```python
from build123d import *

# Parameters (mm, degrees)
PAD007_DEPTH    = 1.5
PAD008_DEPTH    = 0.5
SKETCH012_W     = 5
SKETCH012_H     = 2.5
SKETCH012_W_2   = 7.5
PAD009_DEPTH    = 0.8
SKETCH013_W     = 7.5
SKETCH013_H     = 3
PAD010_DEPTH    = 0.5
POCKET003_DEPTH = 0.5
POCKET004_DEPTH = 2
SKETCH021_W     = 5
SKETCH021_H     = 8
PAD013_DEPTH    = 3.2
SKETCH024_R     = 2.65
POCKET007_DEPTH = 5.201


with BuildPart() as part:
    # Sketch010 → Pad007 (new body)
    with BuildSketch(Plane.XY.offset(-19)):
        with BuildLine():
            Line((-29.25, 13), (29.25, 13))
            ThreePointArc((33, 9.25), (31.9016504294, 11.9016504294), (29.25, 13))
            Line((33, 9.25), (33, -9.25))
            ThreePointArc((29.25, -13), (31.9016504295, -11.9016504294), (33, -9.25))
            Line((29.25, -13), (-29.25, -13))
            ThreePointArc((-33, -9.25), (-31.9016504294, -11.9016504295), (-29.25, -13))
            Line((-33, -9.25), (-33, 9.25))
            ThreePointArc((-29.25, 13), (-31.9016504294, 11.9016504294), (-33, 9.25))
        make_face()
    extrude(amount=PAD007_DEPTH)

    # Sketch011 → Pad008 (new body)
    with BuildSketch(Plane.XY.offset(-17.5)):
        with BuildLine():
            Line((-29.05, 11.3), (29.05, 11.3))
            ThreePointArc((31.3, 9.05), (30.6409902577, 10.6409902577), (29.05, 11.3))
            Line((31.3, 9.05), (31.3, -9.05))
            ThreePointArc((29.05, -11.3), (30.6409902577, -10.6409902577), (31.3, -9.05))
            Line((29.05, -11.3), (-29.05, -11.3))
            ThreePointArc((-31.3, -9.05), (-30.6409902577, -10.6409902577), (-29.05, -11.3))
            Line((-31.3, -9.05), (-31.3, 9.05))
            ThreePointArc((-29.05, 11.3), (-30.6409902577, 10.6409902577), (-31.3, 9.05))
        make_face()
    extrude(amount=PAD008_DEPTH)

    # Sketch012 → Pad009 (new body)
    with BuildSketch(Plane.XY.offset(-17)):
        with Locations((-10.5, 10.55)):
            Rectangle(SKETCH012_W, SKETCH012_H)
        with Locations((10.5, 10.55)):
            Rectangle(SKETCH012_W, SKETCH012_H)
        with Locations((0, -9.75)):
            Rectangle(SKETCH012_W_2, SKETCH012_H)
    extrude(amount=PAD009_DEPTH)

    # Sketch013 → Pad010 (new body)
    with BuildSketch(Plane.XY.offset(-16.2)):
        with Locations((0, -10)):
            Rectangle(SKETCH013_W, SKETCH013_H)
    extrude(amount=PAD010_DEPTH)

    # Sketch016 → Pocket003 (cut)
    with BuildSketch(Plane.XY.offset(-17)):
        with BuildLine():
            ThreePointArc((28.0000015561, -6.5), (26.2322341473, -7.2322319467), (25.5, -8.9999984439))
            ThreePointArc((23.2000163651, -11.3), (24.8263541015, -10.6263414294), (25.5, -8.999998444))
            Line((23.2000163651, -11.5), (23.2000163651, -11.3))
            Line((31.5, -11.5), (23.2000163651, -11.5))
            Line((31.5, -3.2000163651), (31.5, -11.5))
            Line((31.3, -3.2000163651), (31.5, -3.2000163651))
            ThreePointArc((28.0000015561, -6.5), (30.3334480205, -5.5334584921), (31.3, -3.2000163651))
        make_face()
        with BuildLine():
            Line((-23.2000163651, 11.3), (-23.2000163651, 11.5))
            Line((-23.2000163651, 11.5), (-31.5, 11.5))
            Line((-31.5, 11.5), (-31.5, 3.2000163651))
            Line((-31.5, 3.2000163651), (-31.3, 3.2000163651))
            ThreePointArc((-28.000005004, 6.5), (-30.3334514906, 5.5334595241), (-31.3, 3.2000163651))
            ThreePointArc((-28.000005004, 6.5), (-26.2322365854, 7.2322295087), (-25.5, 8.999994996))
            ThreePointArc((-23.2000163651, 11.3), (-24.8263548156, 10.6263397054), (-25.5, 8.999994996))
        make_face()
    extrude(amount=-POCKET003_DEPTH, mode=Mode.SUBTRACT)

    # Sketch017 → Pocket004 (cut)
    with BuildSketch(Plane.XY.offset(-17)):
        with BuildLine():
            ThreePointArc((-24, -6.1), (-25.2, -7.3), (-24, -8.5))
            Line((-24, -8.5), (24, -8.5))
            ThreePointArc((24, -8.5), (25.2, -7.3), (24, -6.1))
            Line((-24, -6.1), (24, -6.1))
        make_face()
    extrude(amount=-POCKET004_DEPTH, mode=Mode.SUBTRACT)

    # Sketch021 → Pad013 (new body)
    with BuildSketch(Plane.XY.offset(-17)):
        with Locations((28.8, 0)):
            Rectangle(SKETCH021_W, SKETCH021_H)
    extrude(amount=PAD013_DEPTH)

    # Sketch024 → Pocket007 (cut, through all)
    with BuildSketch(Plane(origin=(0, 0, -19), x_dir=(1, 0, 0), z_dir=(0, 0, -1))):
        with Locations((-20, -9)):
            Circle(SKETCH024_R)
    extrude(amount=-POCKET007_DEPTH, mode=Mode.SUBTRACT)


solid = part.part
```
Could you check a few things on this model? Use its own coordinates, in mm. A direction names the side the tool comes from. Round coordinates to 2 decimals unless told otherwise and drop trailing zeros. Loops run counter-clockwise (first coordinate to the right, second up) from the corner with the lowest first, then second, coordinate; pieces in that order, holes last. Notation, with made-up numbers: (44.25, -24) - (85.25, -24) arc R17 cw to (85.25, -17) - close; hole circle Ø11 at (-32.75, 88.5). An arc over 180 degrees is marked (long way). Answer in a Markdown table with one row per item. Add a question column.
(1) If we section it at C-C (y = -7.3): Please give me the cut outline in (x, z).
(2) If we mould it in two halves opening along X, with no side actions, what happens to faces 1 (the face through (-26.252, 7.213, -17.246)), 2 (the face through (0, -8.5, -18)), 3 (the face through (0, 13, -18))? For each: pulls with the +X half, pulls with the -X half, needs draft (parallel to the pull), parting line crosses it, or undercut.
(3) I'm going to push flat-ended pins straight in: pin 1 (8 mm diameter, centred on x = 7.5, y = -0.5, fed in from +Z); pin 2 (0.6 mm diameter, centred on x = 1.5, z = -16, fed in from -Y); pin 3 (1 mm diameter, centred on y = -2, z = -16.5, fed in from +X). Where does each tip first touch, or does it pass through?
(4) If we section it at D-D (x = 18): Please give me the cut outline in (y, z), plus the area to 3 significant figures.
(5) If we section it at B-B (x = -20): Please give me the cut outline in (y, z).
(6) If we section it at A-A (x = -11): Please give me the cut outline in (y, z), plus the area to 3 significant figures.
(7) I need wall thicknesses on line 1 along Y through (x, z) = (-20, -17.75); line 2 along X through (y, z) = (9, -17.9); line 3 along Z through (x, y) = (-29, -9). Which ranges of each line are inside material? Lowest first, please.
(8) For faces 4 (the face through (30.66, 10.62, -17.25)), 5 (the face through (-30.66, -10.62, -17.25)), 6 (the face through (24.81, -10.64, -17.25)), which set-ups out of +Z, -Z, +X, -X, +Y, -Y let a thin tool reach every point of the face, with its end or its side?
Model answer:
| question | item | result |
|---|---|---|
| 1 | outline | (-33, -19) - (-25.2, -19) - (-25.2, -17) - (-31.3, -17) - (-31.3, -17.5) - (-33, -17.5) - close; (25.2, -19) - (33, -19) - (33, -17.5) - (26.17, -17.5) - (26.17, -17) - (25.2, -17) - close |
| 2 | face 1 | pulls with the -X half |
| 2 | face 2 | undercut |
| 2 | face 3 | needs draft |
| 3 | pin 1 | stops at z = -17 |
| 3 | pin 2 | stops at y = -11.5 |
| 3 | pin 3 | stops at x = 31.3 |
| 4 | outline | (-13, -19) - (-8.5, -19) - (-8.5, -17) - (-11.3, -17) - (-11.3, -17.5) - (-13, -17.5) - close; (-6.1, -19) - (13, -19) - (13, -17.5) - (11.3, -17.5) - (11.3, -17) - (-6.1, -17) - close |
| 4 | area | 45.5 mm² |
| 5 | outline | (-13, -19) - (-8.5, -19) - (-8.5, -17) - (-11.3, -17) - (-11.3, -17.5) - (-13, -17.5) - close; (-6.1, -19) - (6.35, -19) - (6.35, -17) - (-6.1, -17) - close; (11.65, -19) - (13, -19) - (13, -17.5) - (11.65, -17.5) - close |
| 6 | outline | (-13, -19) - (-8.5, -19) - (-8.5, -17) - (-11.3, -17) - (-11.3, -17.5) - (-13, -17.5) - close; (-6.1, -19) - (13, -19) - (13, -17.5) - (11.3, -17.5) - (11.3, -17) - (11.8, -17) - (11.8, -16.2) - (9.3, -16.2) - (9.3, -17) - (-6.1, -17) - close |
| 6 | area | 47.5 mm² |
| 7 | line 1 | y = -13 to -8.5, -6.1 to 6.35, 11.65 to 13 |
| 7 | line 2 | x = -33 to -22.65, -17.35 to 33 |
| 7 | line 3 | z = -19 to -17 |
| 8 | face 4 | +Z, +X, +Y |
| 8 | face 5 | +Z, -X, -Y |
| 8 | face 6 | +Z, +X, -Y |
